Check sheet for the modelled part. Datum: model origin and axes. Units: mm. A direction names the side the tool comes from. Coordinates: 2 decimals unless noted, no trailing zeros. Loops run counter-clockwise (first coordinate to the right, second up) from the corner with the lowest first, then second, coordinate; pieces in that order, holes last. Notation, with made-up numbers: (81, -17) - (139, -17) arc R14 cw to (139, -6) - close; hole circle Ø8 at (79, -22.5). An arc over 180 degrees is marked (long way). Use a Markdown table: item, result. Add a question column.
1) Go/stop test with flat-tipped pins: P1, Ø1, axis at x = 90.5, z = 29, coming from the -Y side; P2, Ø3, axis at x = 112.5, z = 56.5, coming from the -Y side; P3, Ø24.5, axis at y = 113, z = 0, coming from the -X side. Record where each tip stops, or that it passes through.
2) Thickness scan on line 1 (Y direction, x = 256, z = 0); line 2 (Z direction, x = 245.5, y = 56.5). Record the ranges inside material, lowest first.
3) Tool access check on faces 4 (the conical face through (27.185, 41.186, -9.146)), 5 (the cylindrical face through (251.818, 103.726, 2.059)), 6 (the cylindrical face through (229.37, 92.74, -20.59)). Record the directions out of +Z, -Z, +X, -X, +Y, -Y that give a thin tool (end or side, any length) a straight path to the whole face; none if there is none.
4) Sectioned sample at A-A, the plane z = 0. State how many separate pieces and enclosed holes the cut face has, then the cut area to 3 significant figures.
5) Draft check along Y on faces 1 (the cylindrical face through (106.482, -19.674, 62.475)), 2 (the flat face through (3, 40, 10)), 3 (the cylindrical face through (251.818, -60.139, -106.636)). Enter one of: pulls with the +Y half, pulls with the -Y half, needs draft (parallel to the pull), parting line crosses it, or undercut.
6) Sectioned sample at C-C, the plane y = -113. Enter the section's corners in (x, z), then the cut area to 3 significant figures.
from build123d import *

# Parameters (mm, degrees)
SKETCH_2_R           = 9.5
CUT_EXTRUDE_1_DEPTH  = 321.526909947
SKETCH_3_R           = 9.5
CUT_EXTRUDE_2_DEPTH  = 321.526909947
SKETCH_4_R           = 9.5
CUT_EXTRUDE_3_DEPTH  = 321.526909947
SKETCH_5_R           = 9.5
CUT_EXTRUDE_4_DEPTH  = 321.526909947
SKETCH_6_R           = 9.5
CUT_EXTRUDE_5_DEPTH  = 321.526909947
SKETCH_7_R           = 9.5
CUT_EXTRUDE_6_DEPTH  = 321.526909947
SKETCH_8_R           = 9.5
CUT_EXTRUDE_7_DEPTH  = 321.526909947
SKETCH_9_R           = 9.5
CUT_EXTRUDE_8_DEPTH  = 321.526909947
SKETCH_10_R          = 9.5
CUT_EXTRUDE_9_DEPTH  = 321.526909947
SKETCH_11_R          = 9.5
CUT_EXTRUDE_10_DEPTH = 321.526909947
SKETCH_12_R          = 9.5
CUT_EXTRUDE_11_DEPTH = 321.526909947
SKETCH_13_R          = 9.5
CUT_EXTRUDE_12_DEPTH = 321.526909947


with BuildPart() as part:
    # Эскиз1 → Повернуть1 (revolve)
    with BuildSketch(Plane.XY, mode=Mode.PRIVATE) as revolve_1_sk:
        Polygon((0, 0), (265, 0), (265, 127.5), (239, 127.5), (239, 100), (239, 95), (220, 95), (220, 94), (200, 94), (144, 65.5), (70, 65.5), (25, 41), (3, 41), (3, 45), (0, 45), align=None)
    revolve(revolve_1_sk.sketch.rotate(Axis((0, 0, 0), (1, 0, 0)), 90), axis=Axis((0, 0, 0), (1, 0, 0)))

    # Эскиз2 → Вырез-Вытянуть1 (cut, through all)
    with BuildSketch(Plane(origin=(0, 0, 0), x_dir=(0, 0, -1), z_dir=(1, 0, 0))):
        with Locations((0, 113)):
            Circle(SKETCH_2_R)
    extrude(amount=CUT_EXTRUDE_1_DEPTH, mode=Mode.SUBTRACT)

    # Эскиз3 → Вырез-Вытянуть2 (cut, through all)
    with BuildSketch(Plane(origin=(0, 0, 0), x_dir=(0, 0, -1), z_dir=(1, 0, 0))):
        with Locations((-56.5, 97.860870628)):
            Circle(SKETCH_3_R)
    extrude(amount=CUT_EXTRUDE_2_DEPTH, mode=Mode.SUBTRACT)

    # Эскиз4 → Вырез-Вытянуть3 (cut, through all)
    with BuildSketch(Plane(origin=(0, 0, 0), x_dir=(0, 0, -1), z_dir=(1, 0, 0))):
        with Locations((-97.860870628, 56.5)):
            Circle(SKETCH_4_R)
    extrude(amount=CUT_EXTRUDE_3_DEPTH, mode=Mode.SUBTRACT)

    # Эскиз5 → Вырез-Вытянуть4 (cut, through all)
    with BuildSketch(Plane(origin=(0, 0, 0), x_dir=(0, 0, -1), z_dir=(1, 0, 0))):
        with Locations((-113, 0)):
            Circle(SKETCH_5_R)
    extrude(amount=CUT_EXTRUDE_4_DEPTH, mode=Mode.SUBTRACT)

    # Эскиз6 → Вырез-Вытянуть5 (cut, through all)
    with BuildSketch(Plane(origin=(0, 0, 0), x_dir=(0, 0, -1), z_dir=(1, 0, 0))):
        with Locations((-97.860870628, -56.5)):
            Circle(SKETCH_6_R)
    extrude(amount=CUT_EXTRUDE_5_DEPTH, mode=Mode.SUBTRACT)

    # Эскиз7 → Вырез-Вытянуть6 (cut, through all)
    with BuildSketch(Plane(origin=(0, 0, 0), x_dir=(0, 0, -1), z_dir=(1, 0, 0))):
        with Locations((-56.5, -97.860870628)):
            Circle(SKETCH_7_R)
    extrude(amount=CUT_EXTRUDE_6_DEPTH, mode=Mode.SUBTRACT)

    # Эскиз8 → Вырез-Вытянуть7 (cut, through all)
    with BuildSketch(Plane(origin=(0, 0, 0), x_dir=(0, 0, -1), z_dir=(1, 0, 0))):
        with Locations((0, -113)):
            Circle(SKETCH_8_R)
    extrude(amount=CUT_EXTRUDE_7_DEPTH, mode=Mode.SUBTRACT)

    # Эскиз9 → Вырез-Вытянуть8 (cut, through all)
    with BuildSketch(Plane(origin=(0, 0, 0), x_dir=(0, 0, -1), z_dir=(1, 0, 0))):
        with Locations((56.5, -97.860870628)):
            Circle(SKETCH_9_R)
    extrude(amount=CUT_EXTRUDE_8_DEPTH, mode=Mode.SUBTRACT)

    # Эскиз10 → Вырез-Вытянуть9 (cut, through all)
    with BuildSketch(Plane(origin=(0, 0, 0), x_dir=(0, 0, -1), z_dir=(1, 0, 0))):
        with Locations((97.860870628, -56.5)):
            Circle(SKETCH_10_R)
    extrude(amount=CUT_EXTRUDE_9_DEPTH, mode=Mode.SUBTRACT)

    # Эскиз11 → Вырез-Вытянуть10 (cut, through all)
    with BuildSketch(Plane(origin=(0, 0, 0), x_dir=(0, 0, -1), z_dir=(1, 0, 0))):
        with Locations((113, 0)):
            Circle(SKETCH_11_R)
    extrude(amount=CUT_EXTRUDE_10_DEPTH, mode=Mode.SUBTRACT)

    # Эскиз12 → Вырез-Вытянуть11 (cut, through all)
    with BuildSketch(Plane(origin=(0, 0, 0), x_dir=(0, 0, -1), z_dir=(1, 0, 0))):
        with Locations((97.860870628, 56.5)):
            Circle(SKETCH_12_R)
    extrude(amount=CUT_EXTRUDE_11_DEPTH, mode=Mode.SUBTRACT)

    # Эскиз13 → Вырез-Вытянуть12 (cut, through all)
    with BuildSketch(Plane(origin=(0, 0, 0), x_dir=(0, 0, -1), z_dir=(1, 0, 0))):
        with Locations((56.5, 97.860870628)):
            Circle(SKETCH_13_R)
    extrude(amount=CUT_EXTRUDE_12_DEPTH, mode=Mode.SUBTRACT)


solid = part.part
Solved:
| question | item | result |
|---|---|---|
| 1 | P1 | stops at y = -58.97 |
| 1 | P2 | stops at y = -35.57 |
| 1 | P3 | stops at x = 239 |
| 2 | line 1 | y = -127.5 to -122.5, -103.5 to 103.5, 122.5 to 127.5 |
| 2 | line 2 | z = -114.3 to -107.36, -88.36 to 88.36, 107.36 to 114.3 |
| 3 | face 4 | none |
| 3 | face 5 | +X, -X |
| 3 | face 6 | -X |
| 4 | separate pieces | 3 |
| 4 | enclosed holes | 0 |
| 4 | area | 38,500 mm2 |
| 5 | face 1 | parting line crosses it |
| 5 | face 2 | needs draft |
| 5 | face 3 | undercut |
| 6 | outline | (239, -59.05) - (265, -59.05) - (265, -9.5) - (239, -9.5) - close; (239, 9.5) - (265, 9.5) - (265, 59.05) - (239, 59.05) - close |
| 6 | area | 2,580 mm2 |
